Could you check a few things on this drawing? It's one solid part, dimensions in mm from its lowest x, y, z. A direction names the side the tool comes from. Round coordinates to 2 decimals unless told otherwise and drop trailing zeros. Write each loop counter-clockwise with the first axis right and the second up, starting at its lowest first coordinate (ties: lowest second). Pieces come first, ordered by that corner, then holes. Notation, with made-up numbers: (70.5, 46.5) -> (93.5, 46.5) arc R19 ccw to (93.5, 53.5) -> close; hole circle Ø1 at (7, -28). An arc over 180 degrees is marked (long way). Answer in a Markdown table with one row per item.
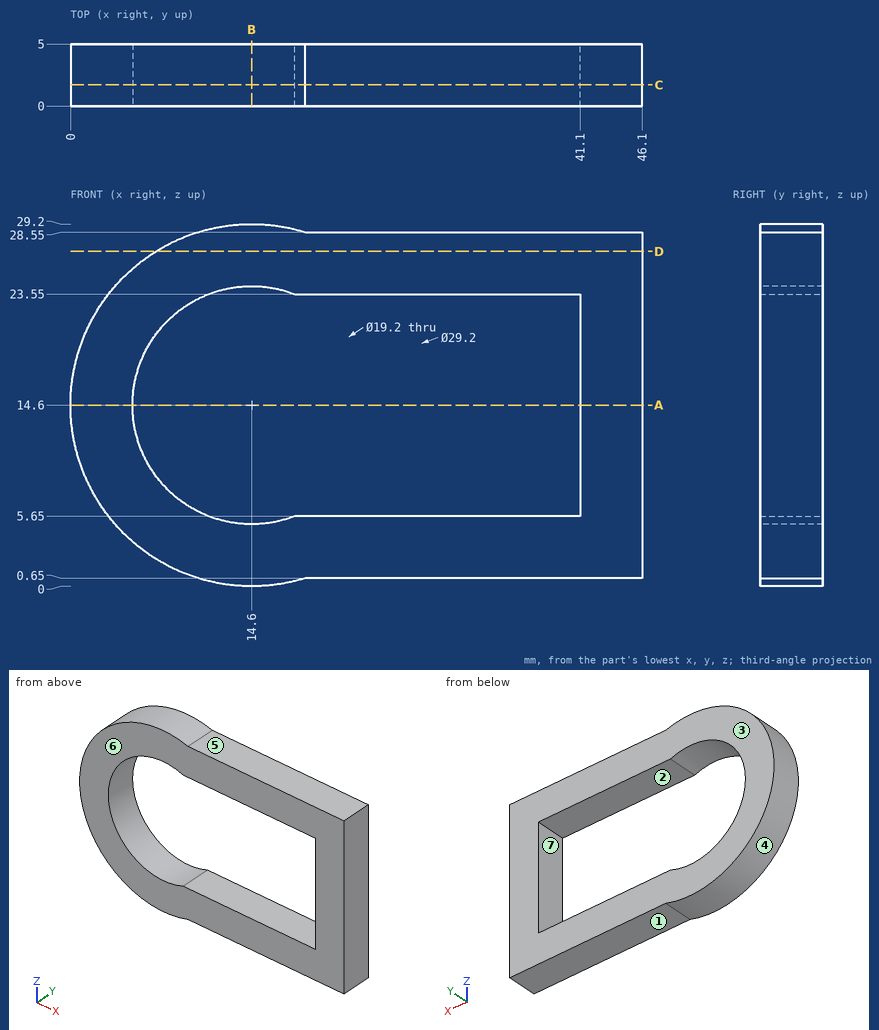
1) Which directions (+Z, -Z, +X, -X, +Y, -Y) give clear straight access to the entire face, cutting with the end or side of a thin tool? Please do the marked faces 5, 6 and 7.
Response:
| item | result |
|---|---|
| face 5 | +Z, +X, +Y, -Y |
| face 6 | +Z, -Z, +X, -X, -Y |
| face 7 | +Y, -Y |
2) I want a section at C-C, the plane y = 1.7. List the corners of the cut face in (x, z) for me.
Response:
| item | result |
|---|---|
| outline | (18.91, 0.65) -> (46.1, 0.65) -> (46.1, 28.55) -> (18.91, 28.55) arc R14.6 ccw (long way) to start; hole (18.07, 5.65) -> (41.1, 5.65) -> (41.1, 23.55) -> (18.07, 23.55) arc R9.6 ccw (long way) to start |
3) For pin 1 (2 mm diameter, centred on x = 18.5, y = 3, fed in from +Z); pin 2 (3 mm diameter, centred on x = 36, y = 2.5, fed in from -Z); pin 3 (2 mm diameter, centred on y = 3, z = 13, fed in from -X); pin 4 (11.5 mm diameter, centred on x = 14.6, z = 14.6, fed in from -Y), each with a flat end and sliding along its axis, tell me the tip position at first contact or that it passes through.
Response:
| item | result |
|---|---|
| pin 1 | stops at z = 28.91 |
| pin 2 | stops at z = 0.65 |
| pin 3 | stops at x = 0.01 |
| pin 4 | passes through |
4) We'd pull the mould along Z, two halves only. Please class the marked faces 1, 2, 3 and 4: +Z half, -Z half, draft (parallel to the pull), parting line (faces both ways), or undercut.
Response:
| item | result |
|---|---|
| face 1 | -Z half |
| face 2 | undercut |
| face 3 | draft |
| face 4 | parting line |
5) I want a section at B-B, the plane x = 14.6. List the corners of the cut face in (y, z) for me.
Response:
| item | result |
|---|---|
| outline | (0, 0) -> (5, 0) -> (5, 5) -> (0, 5) -> close; (0, 24.2) -> (5, 24.2) -> (5, 29.2) -> (0, 29.2) -> close |
6) I want a section at A-A, the plane z = 14.6. List the corners of the cut face in (x, y) for me, and give its area (3 significant figures).
Response:
| item | result |
|---|---|
| outline | (0, 0) -> (5, 0) -> (5, 5) -> (0, 5) -> close; (41.1, 0) -> (46.1, 0) -> (46.1, 5) -> (41.1, 5) -> close |
| area | 50.0 mm^2 |
7) I want a section at D-D, the plane z = 27. List the corners of the cut face in (x, y) for me.
Response:
| item | result |
|---|---|
| outline | (6.89, 0) -> (46.1, 0) -> (46.1, 5) -> (6.89, 5) -> close |
8) I need wall thicknesses on line 1 (Z direction, x = 32.5, y = 3.9); line 2 (Z direction, x = 14.6, y = 2.35); line 3 (X direction, y = 1.15, z = 12.25). Which ranges of each line are inside material? Lowest first, please. Write a range as [from, to].
Response:
| item | result |
|---|---|
| line 1 | z = [0.65, 5.65], [23.55, 28.55] |
| line 2 | z = [0, 5], [24.2, 29.2] |
| line 3 | x = [0.19, 5.29], [41.1, 46.1] |
